```python
from build123d import *

# Parameters (mm, degrees)
SKETCH1_W           = 13.95
SKETCH1_H           = 13.95
BOSS_EXTRUDE1_DEPTH = 6.2


with BuildPart() as part:
    # Sketch1 → Boss-Extrude1 (new body)
    with BuildSketch(Plane(origin=(0, 0, 0), x_dir=(1, 0, 0), z_dir=(0, 1, 0))):
        with BuildLine():
            Line((5, 0), (55.85, 0))
            ThreePointArc((55.85, 0), (57.971320344, -0.878679656), (58.85, -3))
            Line((58.85, -3), (58.85, -42.05))
            ThreePointArc((58.85, -42.05), (57.971320344, -44.171320344), (55.85, -45.05))
            Line((55.85, -45.05), (3, -45.05))
            ThreePointArc((3, -45.05), (0.878679656, -44.171320344), (0, -42.05))
            Line((0, -42.05), (0, -6))
            ThreePointArc((0, -6), (0.292893219, -5.292893219), (1, -5))
            Line((1, -5), (1.1, -5))
            ThreePointArc((1.1, -5), (1.736396103, -4.736396103), (2, -4.1))
            Line((2, -4.1), (2, -3))
            ThreePointArc((2, -3), (2.878679656, -0.878679656), (5, 0))
        make_face()
        with Locations((29.875, -15.175)):
            Rectangle(SKETCH1_W, SKETCH1_H, mode=Mode.SUBTRACT)
        with Locations((10.875, -15.175)):
            Rectangle(SKETCH1_W, SKETCH1_H, mode=Mode.SUBTRACT)
        with Locations((48.875, -15.175)):
            Rectangle(SKETCH1_W, SKETCH1_H, mode=Mode.SUBTRACT)
        with Locations((29.875, -34.175)):
            Rectangle(SKETCH1_W, SKETCH1_H, mode=Mode.SUBTRACT)
        with Locations((48.875, -34.175)):
            Rectangle(SKETCH1_W, SKETCH1_H, mode=Mode.SUBTRACT)
        with Locations((10.875, -34.175)):
            Rectangle(SKETCH1_W, SKETCH1_H, mode=Mode.SUBTRACT)
    extrude(amount=BOSS_EXTRUDE1_DEPTH)


solid = part.part
```
Source: CAD feature listing. Evaluate the final solid. Frame: model axes, mm. A direction names the side the tool comes from. Round coordinates to 2 decimals unless told otherwise and drop trailing zeros. Loops run counter-clockwise (first coordinate to the right, second up) from the corner with the lowest first, then second, coordinate; pieces in that order, holes last. Notation, with made-up numbers: M 24.25,52.25 L 38.25,52.25 A21 ccw 38.25,74.25 Z; hole C -8.5,0 d11. An arc over 180 degrees is marked long. Put each result on its own line as item: value.
(1) Pull-direction query (Z, two-part tool) for faces 1 (the face through (41.9, 3, 15)), 2 (the face through (2.86, 3.06, 0.9)), 3 (the face through (30, 3, 45.05)); classes: released by +Z, released by -Z, zero draft, split by the parting line, or undercut.
Solutions:
face 1: undercut
face 2: released by -Z
face 3: released by +Z
(2) Section C-C, the plane y = 4.25. State how many separate pieces and enclosed holes the cut face has, and give its area (3 significant figures).
Solutions:
separate pieces: 1
enclosed holes: 6
area: 1,470 mm²
(3) Ray query, line 1 (X direction, y = 2, z = 15.5); line 2 (Z direction, x = 8, y = 3.75); line 3 (Z direction, x = 56, y = 5). Return the intervals inside material, ascending. Write a range as [from, to].
Solutions:
line 1: [0, 3.9], [17.85, 22.9], [36.85, 41.9], [55.85, 58.85]
line 2: [0, 8.2], [22.15, 27.2], [41.15, 45.05]
line 3: [0, 45.05]
(4) Access query for faces 4 (the face through (0, 3, 24)), 5 (the face through (3.9, 3, 34)). Directions: +Z, -Z, +X, -X, +Y, -Y. A direction counts if a zero-diameter tool reaches every point of the face in a straight line with its end or side. Return the directions, or none.
Solutions:
face 4: +Z, -Z, -X, +Y, -Y
face 5: +Y, -Y
(5) Section A-A, the plane x = 45. Return loops of the section in (y, z), and give its area (3 significant figures).
Solutions:
outline: M 0,0 L 6.2,0 L 6.2,8.2 L 0,8.2 Z; M 0,22.15 L 6.2,22.15 L 6.2,27.2 L 0,27.2 Z; M 0,41.15 L 6.2,41.15 L 6.2,45.05 L 0,45.05 Z
area: 106 mm²
(6) Section B-B, the plane z = 40. Return loops of the section in (x, y).
Solutions:
outline: M 0,0 L 3.9,0 L 3.9,6.2 L 0,6.2 Z; M 17.85,0 L 22.9,0 L 22.9,6.2 L 17.85,6.2 Z; M 36.85,0 L 41.9,0 L 41.9,6.2 L 36.85,6.2 Z; M 55.85,0 L 58.85,0 L 58.85,6.2 L 55.85,6.2 Z
